Work out the finished part from the listing and answer in its coordinate system (mm). Face numbers are marked on the shaded views. A direction names the side the tool comes from. Round coordinates to 2 decimals unless told otherwise and drop trailing zeros. Order: outer loops, then holes, each group sorted by start corner. A loop starts at its lowest first (then second) coordinate and runs counter-clockwise, first axis right, second up. Notation, with made-up numbers: M 56.5,-35.75 L 86.5,-35.75 A28 cw 86.5,2.25 Z; hole C -20,49.5 d4. An arc over 180 degrees is marked long. Return JSON: item names as keys, results as strings.
from build123d import *

# Parameters (mm, degrees)
CROQUIS2_R                 = 5
CORTAR_EXTRUIR1_DEPTH      = 225.951634778
ESCALA1_SCALE              = 0.8
CORTAR_EXTRUIR2_DEPTH      = 255
CORTAR_EXTRUIR2_DEPTH_BACK = 175
CROQUIS3_W                 = 69.878792472
CROQUIS3_H                 = 224.605431487
CROQUIS5_R                 = 101.510629677
CORTAR_EXTRUIR3_DEPTH      = 1.8
CROQUIS6_R                 = 19.91659092
CORTAR_EXTRUIR4_DEPTH      = 123
CROQUIS7_R                 = 4
CROQUIS7_R_2               = 4.0947051
CORTAR_EXTRUIR5_DEPTH      = 123


with BuildPart() as part:
    # Croquis1 → Revolución1 (revolve)
    with BuildSketch(Plane(origin=(0, 0, 0), x_dir=(1, 0, 0), z_dir=(0, 1, 0)), mode=Mode.PRIVATE) as revoluci_n1_sk:
        Polygon((-84.492307697, 126.907004271), (-84.492307697, 121.907004271), (-77.199679771, 118.257622684), (-61.599944947, 112.544039646), (-54.839043525, 112.544039646), (-54.839043525, 24.920091933), (-36.545776531, 24.920091933), (-36.545776531, 112.544088846), (57.615236657, 112.544088846), (73.214966765, 118.25768476), (80.50759168, 121.907072367), (80.507587553, 126.907072367), (75.507587548, 126.912704348), (75.507589968, 123.980963434), (70.922334115, 123.980959649), (57.615232714, 117.321797618), (-1.992356117, 117.321748418), (-61.599944947, 117.321748418), (-74.907051844, 123.980899465), (-79.492307697, 123.980899465), (-79.492307697, 126.912640379), align=None)
    revolve(revoluci_n1_sk.sketch.rotate(Axis((-84.492307697, 0, 0.092995729), (1, 0, 0)), 180), axis=Axis((-84.492307697, 0, 0.092995729), (1, 0, 0)))

    # Croquis2 → Cortar-Extruir1 (cut, through all)
    with BuildSketch(Plane.ZY.offset(54.839043525)):
        with BuildLine():
            ThreePointArc((30.528582788, -45.440133008), (25.150332276, -46.880047701), (24.664698483, -52.426496358))
            Line((24.664698483, -52.426496358), (34.516411599, -69.490164015))
            ThreePointArc((34.516411599, -69.490164015), (38.954270135, -71.910965134), (43.137091963, -69.072150594))
            Line((43.137091963, -69.072150594), (53.742727711, -55.310992442))
            ThreePointArc((53.742727711, -55.310992442), (54.305907236, -50.480348559), (50.307859812, -47.711249735))
            Line((50.307859812, -47.711249735), (30.528582788, -45.440133008))
        make_face()
        with BuildLine():
            ThreePointArc((45.440133008, 30.528582788), (46.880047701, 25.150332276), (52.426496358, 24.664698483))
            Line((52.426496358, 24.664698483), (69.490164015, 34.516411599))
            ThreePointArc((69.490164015, 34.516411599), (71.910965134, 38.954270135), (69.072150594, 43.137091963))
            Line((69.072150594, 43.137091963), (55.310992442, 53.742727711))
            ThreePointArc((55.310992442, 53.742727711), (50.480348559, 54.305907236), (47.711249735, 50.307859812))
            Line((47.711249735, 50.307859812), (45.440133008, 30.528582788))
        make_face()
        with BuildLine():
            ThreePointArc((-45.440133008, -30.528582788), (-46.880047701, -25.150332276), (-52.426496358, -24.664698483))
            Line((-52.426496358, -24.664698483), (-69.490164015, -34.516411599))
            ThreePointArc((-69.490164015, -34.516411599), (-71.910965134, -38.954270135), (-69.072150594, -43.137091963))
            Line((-69.072150594, -43.137091963), (-55.310992442, -53.742727711))
            ThreePointArc((-55.310992442, -53.742727711), (-50.480348559, -54.305907236), (-47.711249735, -50.307859812))
            Line((-47.711249735, -50.307859812), (-45.440133008, -30.528582788))
        make_face()
        with BuildLine():
            ThreePointArc((-30.528582788, 45.440133008), (-25.150332276, 46.880047701), (-24.664698483, 52.426496358))
            Line((-24.664698483, 52.426496358), (-34.516411599, 69.490164015))
            ThreePointArc((-34.516411599, 69.490164015), (-38.954270135, 71.910965134), (-43.137091963, 69.072150594))
            Line((-43.137091963, 69.072150594), (-53.742727711, 55.310992442))
            ThreePointArc((-53.742727711, 55.310992442), (-54.305907236, 50.480348559), (-50.307859812, 47.711249735))
            Line((-50.307859812, 47.711249735), (-30.528582788, 45.440133008))
        make_face()
        with BuildLine():
            Line((-100.841208128, 17.107848943), (-102.748469547, 0.497407258))
            ThreePointArc((-102.748469547, 0.497407258), (-98.913930395, -4.33194641), (-94.084576727, -0.497407258))
            Line((-94.084576727, -0.497407258), (-92.177315309, 16.113034427))
            ThreePointArc((-92.177315309, 16.113034427), (-96.011854461, 20.942388095), (-100.841208128, 17.107848943))
        make_face()
        with BuildLine():
            Line((17.107848943, 100.841208128), (0.497407258, 102.748469547))
            ThreePointArc((0.497407258, 102.748469547), (-4.33194641, 98.913930395), (-0.497407258, 94.084576727))
            Line((-0.497407258, 94.084576727), (16.113034427, 92.177315309))
            ThreePointArc((16.113034427, 92.177315309), (20.942388095, 96.011854461), (17.107848943, 100.841208128))
        make_face()
        with BuildLine():
            Line((100.841208128, -17.107848943), (102.748469547, -0.497407258))
            ThreePointArc((102.748469547, -0.497407258), (98.913930395, 4.33194641), (94.084576727, 0.497407258))
            Line((94.084576727, 0.497407258), (92.177315309, -16.113034427))
            ThreePointArc((92.177315309, -16.113034427), (96.011854461, -20.942388095), (100.841208128, -17.107848943))
        make_face()
        with BuildLine():
            Line((-17.107848943, -100.841208128), (-0.497407258, -102.748469547))
            ThreePointArc((-0.497407258, -102.748469547), (4.33194641, -98.913930395), (0.497407258, -94.084576727))
            Line((0.497407258, -94.084576727), (-16.113034427, -92.177315309))
            ThreePointArc((-16.113034427, -92.177315309), (-20.942388095, -96.011854461), (-17.107848943, -100.841208128))
        make_face()
        with Locations((50, 0)):
            Circle(CROQUIS2_R)
        with Locations((0, -50)):
            Circle(CROQUIS2_R)
        with Locations((-50, 0)):
            Circle(CROQUIS2_R)
        with Locations((0, 50)):
            Circle(CROQUIS2_R)
    extrude(amount=-CORTAR_EXTRUIR1_DEPTH, mode=Mode.SUBTRACT)


with BuildPart() as part_1:
    # Escala1: scaled about (-24.23364214, 0, 0.097415806)
    add(part.part.scale(ESCALA1_SCALE).moved(Location((-4.846728428, 0, 0.019483161))))

    # Croquis3 → Cortar-Extruir2 (cut, two sides: drawn at the far end of the back side and taken through both)
    with BuildSketch(Plane(origin=(0, 0, 0), x_dir=(1, 0, 0), z_dir=(0, 1, 0)).offset(-CORTAR_EXTRUIR2_DEPTH_BACK)):
        with Locations((34.939396236, -6.332918973)):
            Rectangle(CROQUIS3_W, CROQUIS3_H)
    extrude(amount=CORTAR_EXTRUIR2_DEPTH + CORTAR_EXTRUIR2_DEPTH_BACK, mode=Mode.SUBTRACT)

    # Croquis4 → Revolución3 (revolve)
    with BuildSketch(Plane(origin=(0, 0, 0), x_dir=(1, 0, 0), z_dir=(0, 1, 0))):
        Polygon((0, 93.837921424), (12.264709329, 99.165236946), (15.983101642, 99.165236946), (15.983101642, 101.510629677), (21.767267462, 101.510629677), (21.767267462, 0), (0, 0), align=None)
    revolve(axis=Axis((21.767267462, 0, 0), (-1, 0, 0)))

    # Croquis5 → Cortar-Extruir3 (cut)
    with BuildSketch(Plane(origin=(21.767267462, 0, 0), x_dir=(0, 0, -1), z_dir=(1, 0, 0))):
        Circle(CROQUIS5_R)
    extrude(amount=-CORTAR_EXTRUIR3_DEPTH, mode=Mode.SUBTRACT)

    # Croquis6 → Cortar-Extruir4 (cut)
    with BuildSketch(Plane.ZY.offset(48.717972584)):
        with Locations(Location((0, 0, 0), (0, 0, 180))):
            Circle(CROQUIS6_R)
    extrude(amount=-CORTAR_EXTRUIR4_DEPTH, mode=Mode.SUBTRACT)

    # Croquis7 → Cortar-Extruir5 (cut)
    with BuildSketch(Plane.ZY.offset(48.717972584)):
        with Locations((0.019482626, 40)):
            Circle(CROQUIS7_R)
        with Locations(Location((40.019482626, 0, 0), (0, 0, 180))):
            Circle(CROQUIS7_R_2)
        with Locations((-39.980517374, 0)):
            Circle(CROQUIS7_R)
        with Locations((0.019482626, -40)):
            Circle(CROQUIS7_R)
    extrude(amount=-CORTAR_EXTRUIR5_DEPTH, mode=Mode.SUBTRACT)


solid = part_1.part
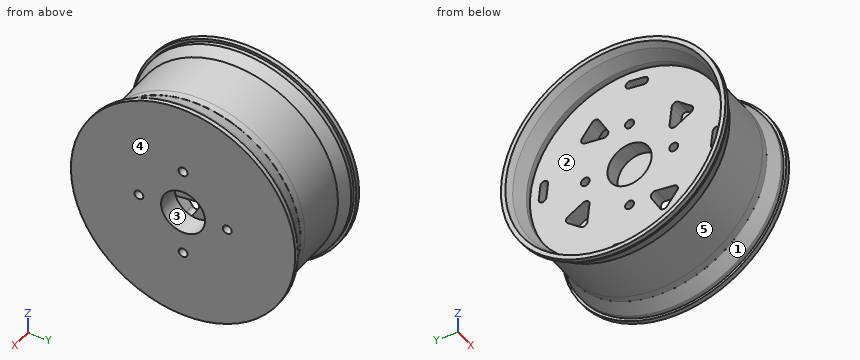
Item 1: The mould has two halves that part along Y. Classify the marked faces 3, 4 and 5: pulls with the +Y half, pulls with the -Y half, needs draft (parallel to the pull), parting line crosses it, or undercut.
Output:
{"face 3": "undercut", "face 4": "needs draft", "face 5": "parting line crosses it"}
Item 2: Each of these flat-tipped pins is pushed along its axis until it touches: pin 1 (9 mm diameter, centred on y = 0, z = -39.98, fed in from -X); pin 2 (5 mm diameter, centred on y = 40, z = 0.02, fed in from -X); pin 3 (2 mm diameter, centred on x = -62.5, z = -80, fed in from -Y); pin 4 (5 mm diameter, centred on x = -16, z = -23.5, fed in from +Y). Where does it stop, or does it pass through?
Output:
{"pin 1": "stops at x = -48.72", "pin 2": "passes through", "pin 3": "stops at y = -58.31", "pin 4": "stops at y = 91.53"}
Item 3: Which of the six approach directions +Z, -Z, +X, -X, +Y, -Y give full straight-line access (tool end or side, diameter ignored) to the marked faces 1 and 2?
Output:
{"face 1": "none", "face 2": "-X"}
Item 4: Find section B-B (x = 4). Determine the outline of the cut face in (y, z).
Output:
{"outline": "C 0,0 d191.15; hole C -40,0.02 d8; hole C 0,0 d39.83; hole C 0,40.02 d8.19; hole C 0,-39.98 d8; hole C 40,0.02 d8"}
Item 5: Find section A-A (x = -30). Determine the outline of the cut face in (y, z).
Output:
{"outline": "C 0,0.09 d187.86; hole C 0,0.09 d180.22"}
Item 6: Consider line 1 along X through (y, z) = (22, -7); line 2 along Y through (x, z) = (-2, 17.5); line 3 along Y through (x, z) = (-56.5, 49). Determine where each line is inside the solid, lowest interval first. Write a range as [from, to].
Output:
{"line 1": "x = [-48.72, -34.08], [0, 19.97]", "line 2": "y = [-92.31, -88.41], [88.41, 92.31]", "line 3": "y = [-81.58, -76.72], [76.72, 81.58]"}
